from build123d import *

# Parameters (mm, degrees)
EXTRUDE1_DEPTH      = 9.525
EXTRUDE1_DEPTH_BACK = 9.525


with BuildPart() as part:
    # Sketch1 → Extrude1 (new, two sides: drawn at the far end of the back side and taken through both)
    with BuildSketch(Plane.XY.offset(-EXTRUDE1_DEPTH_BACK)):
        with BuildLine():
            Line((-0.525296455, -0.092623938), (-0.97555056, -0.172015885))
            ThreePointArc((-0.97555056, -0.172015885), (0.9906, 0), (-0.97555056, 0.172015885))
            Line((-0.97555056, 0.172015885), (-0.525296455, 0.092623938))
            ThreePointArc((-0.525296455, 0.092623938), (0.5334, 0), (-0.525296455, -0.092623938))
        make_face()
    extrude(amount=EXTRUDE1_DEPTH + EXTRUDE1_DEPTH_BACK)

    # Sketch2 → Cut-Revolve1 (revolve, cut)
    with BuildSketch(Plane(origin=(0, 0, 0), x_dir=(0, 0, -1), z_dir=(1, 0, 0))):
        Polygon((9.525, 0.89916), (8.8646, 0.9906), (9.525, 0.9906), align=None)
    cut_revolve1 = revolve(axis=Axis((0, 0, -9.525), (0, 0, 1)), mode=Mode.SUBTRACT)

    # Mirror1: Cut-Revolve1 across plane
    add(cut_revolve1.mirror(Plane.XY), mode=Mode.SUBTRACT)


solid = part.part
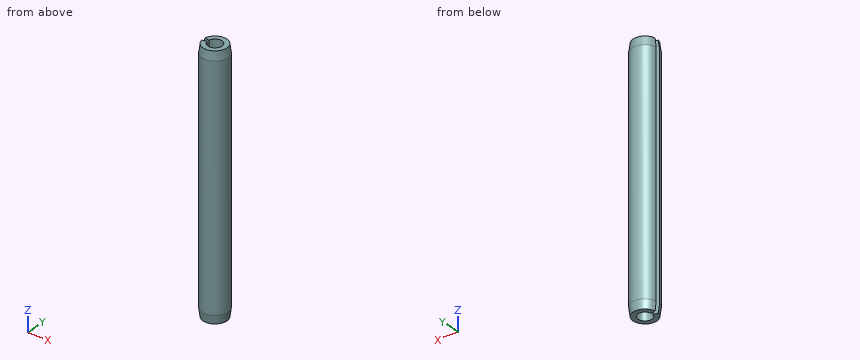
Could you check a few things on this model? Use its own coordinates, in mm. Coordinates: 2 decimals unless noted, no trailing zeros. Order: outer loops, then holes, each group sorted by start corner. A loop starts at its lowest first (then second) coordinate and runs counter-clockwise, first axis right, second up.
Q1. Suppose I cut it at A-A on x = 0. Please give me the cut outline in (y, z) (3 decimals), and give its area (3 significant figures).
Q2. Please list where these lines run through material, in increasing order: L1, parallel to Y at x = 0, z = -5.5; L2, parallel to X at y = -0.05, z = 6.75; L3, parallel to X at y = 0.45, z = 7.25.
Q3. Suppose I cut it at B-B on z = -1.25. Please give me the cut outline in (x, y).
Answer:
1. outline: (-0.991, -8.865) - (-0.899, -9.525) - (-0.533, -9.525) - (-0.533, 9.525) - (-0.899, 9.525) - (-0.991, 8.865) - close; (0.533, -9.525) - (0.899, -9.525) - (0.991, -8.865) - (0.991, 8.865) - (0.899, 9.525) - (0.533, 9.525) - close
1. area: 17.3 mm2
2. L1: y = -0.99 to -0.53, 0.53 to 0.99
2. L2: x = 0.53 to 0.99
2. L3: x = -0.88 to -0.29, 0.29 to 0.88
3. outline: (-0.98, -0.17) arc R0.99 ccw (long way) to (-0.98, 0.17) - (-0.53, 0.09) arc R0.53 cw (long way) to (-0.53, -0.09) - close
